Geometry check sheet. Reference: the model listing, model coordinates, mm. Give positions to 0.01 mm unless a question says otherwise; leave off trailing zeros. Order: outer loops, then holes, each group sorted by start corner. A loop starts at its lowest first (then second) coordinate and runs counter-clockwise, first axis right, second up. Notation, with made-up numbers: M 47,-21.5 L 65,-21.5 A28 ccw 65,9.5 Z; hole C 81,26.5 d6. An arc over 180 degrees is marked long. Use CSV: the item, a comma, the result in double quotes. Start each with the question number.
from build123d import *

# Parameters (mm, degrees)
SKETCH1_W           = 150
SKETCH1_H           = 140
SKETCH1_R           = 9
BOSS_EXTRUDE1_DEPTH = 10


with BuildPart() as part:
    # Sketch1 → Boss-Extrude1 (new body)
    with BuildSketch(Plane.XY.offset(10)):
        Rectangle(SKETCH1_W, SKETCH1_H)
        with Locations(Location((-17.5, -22, 0), (0, 0, 180))):
            Circle(SKETCH1_R, mode=Mode.SUBTRACT)
        with Locations(Location((-45.5, -22, 0), (0, 0, 180))):
            Circle(SKETCH1_R, mode=Mode.SUBTRACT)
        with Locations(Location((10.5, -22, 0), (0, 0, 180))):
            Circle(SKETCH1_R, mode=Mode.SUBTRACT)
        with Locations(Location((38.5, -22, 0), (0, 0, 180))):
            Circle(SKETCH1_R, mode=Mode.SUBTRACT)
        with Locations(Location((-45.5, 6, 0), (0, 0, 180))):
            Circle(SKETCH1_R, mode=Mode.SUBTRACT)
        with Locations(Location((-17.5, 6, 0), (0, 0, 180))):
            Circle(SKETCH1_R, mode=Mode.SUBTRACT)
        with Locations(Location((10.5, 6, 0), (0, 0, 180))):
            Circle(SKETCH1_R, mode=Mode.SUBTRACT)
        with Locations(Location((38.5, 6, 0), (0, 0, 180))):
            Circle(SKETCH1_R, mode=Mode.SUBTRACT)
        with Locations(Location((-45.5, 34, 0), (0, 0, 180))):
            Circle(SKETCH1_R, mode=Mode.SUBTRACT)
        with Locations(Location((-17.5, 34, 0), (0, 0, 180))):
            Circle(SKETCH1_R, mode=Mode.SUBTRACT)
        with Locations(Location((10.5, 34, 0), (0, 0, 180))):
            Circle(SKETCH1_R, mode=Mode.SUBTRACT)
        with Locations(Location((38.5, 34, 0), (0, 0, 180))):
            Circle(SKETCH1_R, mode=Mode.SUBTRACT)
    extrude(amount=-BOSS_EXTRUDE1_DEPTH)


solid = part.part
(1) Sectioned sample at B-B on y = 34. Record the cut outline in (x, z).
(2) Sectioned sample at A-A on x = -45.5. Record the cut outline in (y, z), then the cut area to 3 significant figures.
(3) Sectioned sample at D-D on x = 16. Record the cut outline in (y, z).
(4) Thickness scan on line 1 (Y direction, x = 38.5, z = 4.75); line 2 (X direction, y = 34, z = 2.5); line 3 (Y direction, x = 5, z = 4.5). Record the ranges inside material, lowest first.
(5) Go/stop test with a flat-tipped pin: P1, Ø16, axis at x = 38.5, y = 6, coming from the +Z side. Record where the tip stops, or that it passes through.
(6) Sectioned sample at C-C on z = 4.5. Give the number of separate pieces and of enclosed holes in the cut face, then the cut area to 3 significant figures.
Responses:
1,outline,"M -75,0 L -54.5,0 L -54.5,10 L -75,10 Z; M -36.5,0 L -26.5,0 L -26.5,10 L -36.5,10 Z; M -8.5,0 L 1.5,0 L 1.5,10 L -8.5,10 Z; M 19.5,0 L 29.5,0 L 29.5,10 L 19.5,10 Z; M 47.5,0 L 75,0 L 75,10 L 47.5,10 Z"
2,outline,"M -70,0 L -31,0 L -31,10 L -70,10 Z; M -13,0 L -3,0 L -3,10 L -13,10 Z; M 15,0 L 25,0 L 25,10 L 15,10 Z; M 43,0 L 70,0 L 70,10 L 43,10 Z"
2,area,"860 mm2"
3,outline,"M -70,0 L -29.12,0 L -29.12,10 L -70,10 Z; M -14.88,0 L -1.12,0 L -1.12,10 L -14.88,10 Z; M 13.12,0 L 26.88,0 L 26.88,10 L 13.12,10 Z; M 41.12,0 L 70,0 L 70,10 L 41.12,10 Z"
4,line 1,"-70 to -31, -13 to -3, 15 to 25, 43 to 70"
4,line 2,"-75 to -54.5, -36.5 to -26.5, -8.5 to 1.5, 19.5 to 29.5, 47.5 to 75"
4,line 3,"-70 to -29.12, -14.88 to -1.12, 13.12 to 26.88, 41.12 to 70"
5,P1,"through"
6,separate pieces,"1"
6,enclosed holes,"12"
6,area,"17,900 mm2"
